Source: CAD feature listing. Evaluate the final solid. Frame: model axes, mm. Round coordinates to 2 decimals unless told otherwise and drop trailing zeros. Order: outer loops, then holes, each group sorted by start corner. A loop starts at its lowest first (then second) coordinate and runs counter-clockwise, first axis right, second up.
Autodesk Inventor part; units mm, degrees
ref_plane "YZ Plane" through (0, 0, 0) normal (1, 0, 0) x (0, 1, 0)
ref_plane "XZ Plane" through (0, 0, 0) normal (0, 1, 0) x (-1, 0, 0)
ref_plane "XY Plane" through (0, 0, 0) normal (0, 0, 1) x (1, 0, 0)
sketch "Szkic3" plane through (0, 0, 0) normal (0, 1, 0) x (-1, 0, 0)
  line L0 (0, 0) -> (-20, 0)
  line L1 (-20, 0) -> (-20, -20)
  line L2 (-20, -20) -> (0, -20)
  line L3 (0, -20) -> (0, 0)
  dimension "d6" = 20
  dimension "d7" = 20
extrude "Wyciągnięcie proste3" add sketch "Szkic3" along normal blind 5
sketch "Szkic4" plane through (0, 0, 0) normal (0, -1, 0) x (1, 0, 0)
  line L0 (0, 0) -> (20, 0)
  line L1 (20, 0) -> (20, -20)
  line L2 (0, 0) -> (20, -20)
  line L3 (20, -20) -> (20, 0)
  line L4 (20, 0) -> (0, 0)
extrude "Wyciągnięcie proste4" cut sketch "Szkic4" against normal blind 5
sketch "Szkic5" plane through (0, 5, 0) normal (0, 1, 0) x (1, 0, 0)
  line L0 (0, 20) -> (0, 0)
  line L1 (0, 20) -> (10.5726, 9.4274)
  line L2 (0, 0) -> (20, 20)
  line L3 (10.5726, 9.4274) -> (0, -1.1451)
  line L4 (20, 20) -> (0, 20)
  line L5 (0, -1.1451) -> (0, 20)
  point P0 (10, 10)
extrude "Wyciągnięcie proste5" cut sketch "Szkic5" against normal blind 10 contours L1 L2 L0
properties part number "Helenowiak_podpora"
1. Section C-C on y = 3.75. Return loops of the section in (x, z), plus the area to 3 significant figures.
2. Line query: line 1 along X through (y, z) = (4, -13); line 2 along Z through (x, y) = (17.25, 1.55); line 3 along Z through (x, y) = (4.5, 3.45). Output: solid intervals per line, ascending.
3. Section B-B on z = -12. Return loops of the section in (x, y).
4. First-contact query: pin 1 (1 mm diameter, centred on y = 1.5, z = -16, fed in from -X); pin 2 (3 mm diameter, centred on x = 2.5, y = 2, fed in from +Z); pin 3 (6 mm diameter, centred on x = 6.5, z = -12, fed in from -Y). Flat tips, straight axial feed; report the tip coordinate or a pass-through.
5. Section A-A on x = 4.25. Return loops of the section in (y, z).
Result:
1. outline: (0, -20) - (20, -20) - (10, -10) - close
1. area: 100 mm2
2. line 1: x = 7 to 13
2. line 2: z = -20 to -17.25
2. line 3: z = -20 to -15.5
3. outline: (8, 0) - (12, 0) - (12, 5) - (8, 5) - close
4. pin 1: stops at x = 3.5
4. pin 2: stops at z = -16
4. pin 3: stops at y = 0
5. outline: (0, -20) - (5, -20) - (5, -15.75) - (0, -15.75) - close
